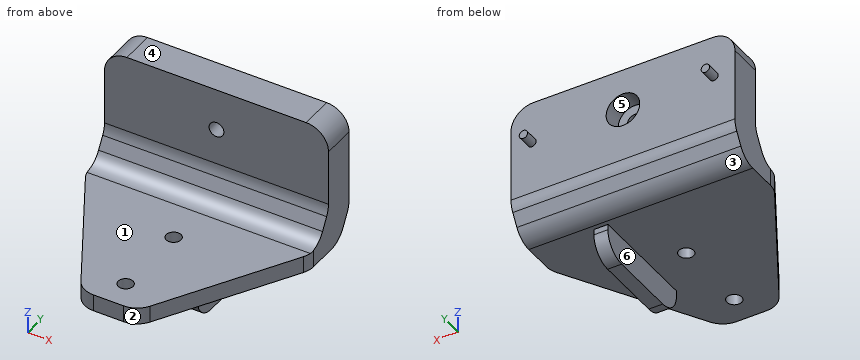
```python
from build123d import *
from OCP.BRepFilletAPI import BRepFilletAPI_MakeChamfer

# Parameters (mm, degrees)
BOSS_EXTRUDE1_DEPTH = 40
SKETCH2_R           = 2.65
CUT_EXTRUDE2_DEPTH  = 12
SKETCH3_R           = 6
CUT_EXTRUDE3_DEPTH  = 7
CUT_EXTRUDE4_REACH  = 86.67
SKETCH4_R           = 2.65
CHAMFER2_SIZE       = 30
CHAMFER2_SIZE2      = 51.961524227
SKETCH7_W           = 5
SKETCH7_H           = 40
BOSS_EXTRUDE3_DEPTH = 10
CHAMFER1_SIZE       = 10
CHAMFER1_SIZE2      = 5.773502692
FILLET1_R           = 8
FILLET2_R           = 8
SKETCH5_R           = 1.5
BOSS_EXTRUDE2_DEPTH = 5
FILLET3_R           = 8


with BuildPart() as part:
    # Sketch1 → Boss-Extrude1 (new, symmetric)
    with BuildSketch(Plane(origin=(0, 0, 0), x_dir=(0, 0, -1), z_dir=(1, 0, 0))):
        Polygon((0, 0), (40, 0), (40, -63), (46, -63), (46, 12), (0, 12), align=None)
    extrude(amount=BOSS_EXTRUDE1_DEPTH, both=True)

    # Sketch2 → Cut-Extrude2 (cut)
    with BuildSketch(Plane.XZ):
        with Locations(Location((0, -15, 0), (0, 0, 270))):
            Circle(SKETCH2_R)
    extrude(amount=-CUT_EXTRUDE2_DEPTH, mode=Mode.SUBTRACT)

    # Sketch3 → Cut-Extrude3 (cut)
    with BuildSketch(Plane(origin=(0, 12, 0), x_dir=(1, 0, 0), z_dir=(0, 1, 0))):
        with Locations(Location((0, 15, 0), (0, 0, 270))):
            Circle(SKETCH3_R)
    extrude(amount=-CUT_EXTRUDE3_DEPTH, mode=Mode.SUBTRACT)

    # Sketch4 → Cut-Extrude4 (cut, up to next)
    with BuildSketch(Plane.XY.offset(-40), mode=Mode.PRIVATE) as cut_extrude4_sk1:
        with Locations((0, -53)):
            Circle(SKETCH4_R)
    cut_extrude4_tool1 = extrude(cut_extrude4_sk1.sketch, amount=-CUT_EXTRUDE4_REACH, mode=Mode.PRIVATE) & part.part
    # Sketch4 → Cut-Extrude4 (cut, up to next)
    with BuildSketch(Plane.XY.offset(-40), mode=Mode.PRIVATE) as cut_extrude4_sk2:
        with Locations((0, -25)):
            Circle(SKETCH4_R)
    cut_extrude4_tool2 = extrude(cut_extrude4_sk2.sketch, amount=-CUT_EXTRUDE4_REACH, mode=Mode.PRIVATE) & part.part
    add(cut_extrude4_tool1.solids().sort_by_distance((0, -53, -40))[0], mode=Mode.SUBTRACT)
    add(cut_extrude4_tool2.solids().sort_by_distance((0, -25, -40))[0], mode=Mode.SUBTRACT)

    # Chamfer2
    chamfer2_edges = [part.edges().sort_by_distance(p)[0] for p in [
        (40, -63, -43),
        (-40, -63, -43),
    ]]
    chamfer2_side = [part.faces().sort_by_distance(p)[0] for p in [
        (0, -63, -43),
    ]]
    chamfer(chamfer2_edges, length=CHAMFER2_SIZE, length2=CHAMFER2_SIZE2, reference=chamfer2_side[0])

    # Sketch7 → Boss-Extrude3 (add)
    with BuildSketch(Plane(origin=(0, 0, -46), x_dir=(-1, 0, 0), z_dir=(0, 0, -1))):
        with Locations((-15.2, -20)):
            Rectangle(SKETCH7_W, SKETCH7_H)
    extrude(amount=BOSS_EXTRUDE3_DEPTH)

    # Chamfer1: one chamfer whose edges measure the first distance from different faces: ONE call of the kernel's chamfer builder (chamfer() names one face for all edges)
    chamfer1_edges_1 = [part.edges().sort_by_distance(p)[0] for p in [
        (0, 12, -46),
    ]]
    chamfer1_side_1 = [part.faces().sort_by_distance(p)[0] for p in [
        (0, 12, -23.253659483),
    ]]
    chamfer1_edges_2 = [part.edges().sort_by_distance(p)[0] for p in [
        (0, 0, -40),
    ]]
    chamfer1_side_2 = [part.faces().sort_by_distance(p)[0] for p in [
        (0, 0, -20.034710925),
    ]]
    chamfer1 = BRepFilletAPI_MakeChamfer(part.part.solid().wrapped)
    for e in chamfer1_edges_1:
        chamfer1.Add(CHAMFER1_SIZE, CHAMFER1_SIZE2, e.wrapped, chamfer1_side_1[0].wrapped)  # the first distance lies on this face
    for e in chamfer1_edges_2:
        chamfer1.Add(CHAMFER1_SIZE, CHAMFER1_SIZE2, e.wrapped, chamfer1_side_2[0].wrapped)  # the first distance lies on this face
    add(Compound.cast(chamfer1.Shape()), mode=Mode.REPLACE)

    # Fillet1
    fillet1_edges = [part.edges().sort_by_distance(p)[0] for p in [
        (0, 12, -36),
        (0, 6.226497308, -46),
        (0, -5.773502692, -40),
        (0, 0, -30),
    ]]
    fillet(fillet1_edges, radius=FILLET1_R)

    # Fillet2
    fillet2_edges = [part.edges().sort_by_distance(p)[0] for p in [
        (-40, 6, 0),
        (40, 6, 0),
        (-40, -11.038475773, -43),
        (40, -11.038475773, -43),
        (10, -63, -43),
        (-10, -63, -43),
    ]]
    fillet(fillet2_edges, radius=FILLET2_R)

    # Sketch5 → Boss-Extrude2 (add)
    with BuildSketch(Plane(origin=(0, 12, 0), x_dir=(1, 0, 0), z_dir=(0, 1, 0))):
        with Locations(Location((-32.5, 15, 0), (0, 0, 90))):
            Circle(SKETCH5_R)
        with Locations(Location((32.5, 15, 0), (0, 0, 90))):
            Circle(SKETCH5_R)
    extrude(amount=BOSS_EXTRUDE2_DEPTH)

    # Fillet3
    fillet3_edges = [part.edges().sort_by_distance(p)[0] for p in [
        (15.2, 0, -56),
        (15.2, -40, -56),
    ]]
    fillet(fillet3_edges, radius=FILLET3_R)


solid = part.part
```
Design review of the part built by this model. Coordinates are the model's own, in mm. Face numbers are marked on the shaded views. A direction names the side the tool comes from. Coordinates: 2 decimals unless noted, no trailing zeros. Loops run counter-clockwise (first coordinate to the right, second up) from the corner with the lowest first, then second, coordinate; pieces in that order, holes last.
Q1. We need section C-C on y = -53. State the section outline as (x, z) points, and give its area (3 significant figures).
Reported:
outline: (-15.77, -46) - (-2.65, -46) - (-2.65, -40) - (-15.77, -40) - close; (2.65, -46) - (15.77, -46) - (15.77, -40) - (2.65, -40) - close
area: 157 mm2
Q2. Tool access review of the marked faces 1 and 2: name each direction out of +Z, -Z, +X, -X, +Y, -Y from which nothing blocks a thin tool from reaching the whole face with its end or side.
Reported:
face 1: +Z, +X, -X, -Y
face 2: +Z, -Z, +X, -Y
Q3. We need section A-A on x = 0. State the section outline as (y, z) points.
Reported:
outline: (-63, -46) - (-55.65, -46) - (-55.65, -40) - (-63, -40) - close; (-50.35, -46) - (-27.65, -46) - (-27.65, -40) - (-50.35, -40) - close; (-22.35, -46) - (1.61, -46) arc R8 ccw to (8.54, -42) - (10.93, -37.86) arc R8 ccw to (12, -33.86) - (12, -21) - (5, -21) - (5, -17.65) - (0, -17.65) - (0, -27.86) arc R8 cw to (-1.07, -31.86) - (-3.46, -36) arc R8 cw to (-10.39, -40) - (-22.35, -40) - close; (0, -12.35) - (5, -12.35) - (5, -9) - (12, -9) - (12, 0) - (0, 0) - close
Q4. The part is to be moulded in two halves that separate along Z. For the marked faces 3, 4, 5 and 6, say which applies: +Z half, -Z half, draft (parallel to the pull), parting line (faces both ways), or undercut.
Reported:
face 3: -Z half
face 4: +Z half
face 5: undercut
face 6: draft
Q5. We need section D-D on y = -17. State the section outline as (x, z) points.
Reported:
outline: (-36.56, -46) - (12.7, -46) - (12.7, -56) - (17.7, -56) - (17.7, -46) - (36.56, -46) - (36.56, -40) - (-36.56, -40) - close
Q6. For pin 1 (3 mm diameter, centred on y = -8, z = -49.5, fed in from +X); pin 2 (3 mm diameter, centred on x = 0, y = -25, fed in from -Z); pin 3 (8 mm diameter, centred on x = -20, z = -15.5, fed in from -Y); pin 4 (4 mm diameter, centred on y = -25.5, z = -45, fed in from +X), all flat-tipped, find the tip position at first contact; note any pin that passes through.
Reported:
pin 1: stops at x = 17.7
pin 2: passes through
pin 3: stops at y = 0
pin 4: stops at x = 32.81
Q7. We need section B-B on z = -15. State the section outline as (x, y) points, and give its area (4 significant figures).
Reported:
outline: (-40, 0) - (-2.65, 0) - (-2.65, 5) - (-6, 5) - (-6, 12) - (-31, 12) - (-31, 17) - (-34, 17) - (-34, 12) - (-40, 12) - close; (2.65, 0) - (40, 0) - (40, 12) - (34, 12) - (34, 17) - (31, 17) - (31, 12) - (6, 12) - (6, 5) - (2.65, 5) - close
area: 879.5 mm2
Q8. To check wall thickness, follow line 1 (Y direction, x = 0, z = -44.7); line 2 (X direction, y = 1.4, z = -15); line 3 (X direction, y = 8, z = -15). State the ranges of each line that lie inside material, in increasing order.
Reported:
line 1: y = -63 to -55.65, -50.35 to -27.65, -22.35 to 5.98
line 2: x = -40 to -2.65, 2.65 to 40
line 3: x = -40 to -6, 6 to 40
